Could you check a few things on this model? Use its own coordinates, in mm. Face numbers are marked on the shaded views. A direction names the side the tool comes from. Round coordinates to 2 decimals unless told otherwise and drop trailing zeros. Write each loop counter-clockwise with the first axis right and the second up, starting at its lowest first coordinate (ties: lowest second). Pieces come first, ordered by that corner, then holes. Notation, with made-up numbers: M 89.25,-35 L 122.25,-35 A18 cw 122.25,-10 Z; hole C -31,41.5 d4. An arc over 180 degrees is marked long. One line per item, written item: value. Start each with the question number.
(1) If I drill on L1, parallel to X at y = -26, z = 42.5; L2, parallel to X at y = -22, z = 8; L3, parallel to Z at x = -36, y = -35, over which ranges is the centre line in solid material (lowest first)?
(2) Thinking about a two-plate mould opening in Z: for the marked faces 1, 2, 3 and 4, which applies, released by +Z, released by -Z, zero draft, split by the parting line, or undercut?
(3) I want a section at C-C on z = -29.5. Please give me the cut outline in (x, y), and give its area (3 significant figures).
(4) I want a section at A-A on z = 0. Please give me the cut outline in (x, y).
(5) I want a section at B-B on x = -30. Please give me the cut outline in (y, z), and give its area (3 significant figures).
(6) I'm going to push flat-ended pins straight in: pin 1 Ø6 at (y, z) = (-21.5, 3) entering from -X; pin 2 Ø10 at (x, y) = (-27.5, -72) entering from -Z; pin 3 Ø4 at (x, z) = (-33, 17.5) entering from +Y. Where does each tip first touch, or does it pass through?
(7) Which directions (+Z, -Z, +X, -X, +Y, -Y) give clear straight access to the entire face, cutting with the end or side of a thin tool? Please do the marked faces 5, 6 and 7.
(8) I want a section at D-D on x = -3. Please give me the cut outline in (y, z).
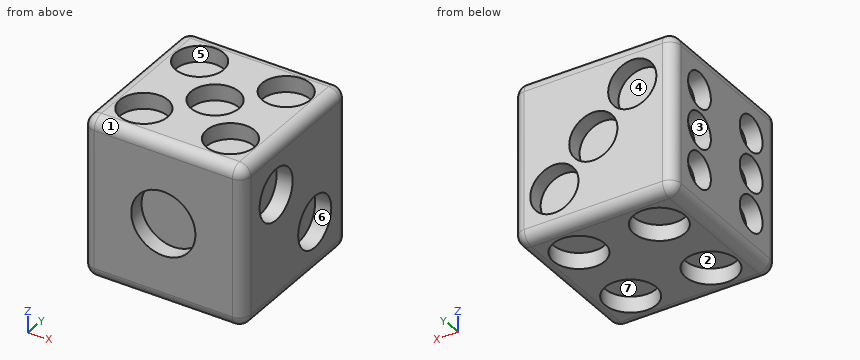
```python
from build123d import *

# Parameters (mm, degrees)
F0_W      = 100
F0_H      = 100
F1_DEPTH  = 100
F3_R      = 20
F4_DEPTH  = 10
F5_R      = 15
F6_DEPTH  = 10
F7_R      = 16
F8_DEPTH  = 10
F2_R      = 16
F9_DEPTH  = 10
F10_R     = 11
F11_DEPTH = 10
F12_R     = 15
F13_DEPTH = 10
F14_R     = 7


with BuildPart() as f1:
    # F0 (on Front) → F1 (new body)
    with BuildSketch(Plane.XZ):
        Rectangle(F0_W, F0_H)
    extrude(amount=F1_DEPTH)

    # F3 (on face) → F4 (cut)
    with BuildSketch(Plane.XZ.offset(100)):
        Circle(F3_R)
    extrude(amount=-F4_DEPTH, mode=Mode.SUBTRACT)

    # F5 (on face) → F6 (cut)
    with BuildSketch(Plane.XY.offset(50)):
        with Locations((-26.872959, -77.044369)):
            Circle(F5_R)
        with Locations((27.032832, -77.044369)):
            Circle(F5_R)
        with Locations((27.032832, -23.138578)):
            Circle(F5_R)
        with Locations((-26.872959, -23.138578)):
            Circle(F5_R)
        with Locations((0.079937, -50.091474)):
            Circle(F5_R)
    extrude(amount=-F6_DEPTH, mode=Mode.SUBTRACT)

    # F7 (on face) → F8 (cut)
    with BuildSketch(Plane(origin=(0, 0, -50), x_dir=(1, 0, 0), z_dir=(0, 0, -1))):
        with Locations((-25, 75)):
            Circle(F7_R)
        with Locations((25, 75)):
            Circle(F7_R)
        with Locations((25, 25)):
            Circle(F7_R)
        with Locations((-25, 25)):
            Circle(F7_R)
    extrude(amount=-F8_DEPTH, mode=Mode.SUBTRACT)

    # F2 (on face) → F9 (cut)
    with BuildSketch(Plane.YZ.offset(50)):
        with Locations((-68.583503, 18.583503)):
            Circle(F2_R)
        with Locations((-31.224914, -18.775086)):
            Circle(F2_R)
    extrude(amount=-F9_DEPTH, mode=Mode.SUBTRACT)

    # F10 (on face) → F11 (cut)
    with BuildSketch(Plane(origin=(-50, 0, 0), x_dir=(0, -1, 0), z_dir=(-1, 0, 0))):
        with Locations((25, 25)):
            Circle(F10_R)
        with Locations((25, 0)):
            Circle(F10_R)
        with Locations((25, -25)):
            Circle(F10_R)
        with Locations((75, -25)):
            Circle(F10_R)
        with Locations((75, 0)):
            Circle(F10_R)
        with Locations((75, 25)):
            Circle(F10_R)
    extrude(amount=-F11_DEPTH, mode=Mode.SUBTRACT)

    # F12 (on face) → F13 (cut)
    with BuildSketch(Plane.XZ):
        Circle(F12_R)
        with Locations((-24.242424, 24.242424)):
            Circle(F12_R)
        with Locations((24.242424, -24.242424)):
            Circle(F12_R)
    extrude(amount=F13_DEPTH, mode=Mode.SUBTRACT)

    # F14
    f14_edges = [f1.edges().sort_by_distance(p)[0] for p in [
        (-50, -50, 50),
        (0, -100, -50),
        (0, -100, 50),
        (-50, -100, 0),
        (50, -100, 0),
        (50, -50, -50),
        (50, 0, 0),
        (50, -50, 50),
        (0, 0, 50),
        (0, 0, -50),
        (-50, 0, 0),
        (-50, -50, -50),
    ]]
    fillet(f14_edges, radius=F14_R)


solid = f1.part
```
Found:
1. L1: x = -50 to -41.6, -12.15 to 12.31, 41.76 to 50
1. L2: x = -40 to 50
1. L3: z = -40 to 40
2. face 1: released by +Z
2. face 2: released by -Z
2. face 3: undercut
2. face 4: undercut
3. outline: M -50,-93 A7 ccw -43,-100 L 43,-100 A7 ccw 50,-93 L 50,-43.1 L 40,-43.1 L 40,-19.35 L 50,-19.35 L 50,-7 A7 ccw 43,0 L 38.29,0 L 38.29,-10 L 10.19,-10 L 10.19,0 L -43,0 A7 ccw -50,-7 L -50,-14.96 L -40,-14.96 L -40,-35.04 L -50,-35.04 L -50,-64.96 L -40,-64.96 L -40,-85.04 L -50,-85.04 Z
3. area: 9,040 mm²
4. outline: M -50,-93 A7 ccw -43,-100 L -20,-100 L -20,-90 L 20,-90 L 20,-100 L 43,-100 A7 ccw 50,-93 L 50,-7 A7 ccw 43,0 L 15,0 L 15,-10 L -15,-10 L -15,0 L -43,0 A7 ccw -50,-7 L -50,-14 L -40,-14 L -40,-36 L -50,-36 L -50,-64 L -40,-64 L -40,-86 L -50,-86 Z
5. outline: M -100,-43 A7 ccw -93,-50 L -90.2,-50 L -90.2,-40 L -59.8,-40 L -59.8,-50 L -40.2,-50 L -40.2,-40 L -9.8,-40 L -9.8,-50 L -7,-50 A7 ccw 0,-43 L 0,10.39 L -10,10.39 L -10,38.09 L 0,38.09 L 0,43 A7 ccw -7,50 L -8.47,50 L -8.47,40 L -37.81,40 L -37.81,50 L -62.37,50 L -62.37,40 L -91.71,40 L -91.71,50 L -93,50 A7 ccw -100,43 Z
5. area: 8,490 mm²
6. pin 1: stops at x = -40
6. pin 2: stops at z = -40
6. pin 3: stops at y = -10
7. face 5: +Z
7. face 6: +X
7. face 7: -Z
8. outline: M -100,-43 A7 ccw -93,-50 L -7,-50 A7 ccw 0,-43 L 0,-14.7 L -10,-14.7 L -10,14.7 L 0,14.7 L 0,43 A7 ccw -7,50 L -35.41,50 L -35.41,40 L -64.77,40 L -64.77,50 L -93,50 A7 ccw -100,43 L -100,19.77 L -90,19.77 L -90,-19.77 L -100,-19.77 Z
